Autodesk Inventor part; units mm, degrees
ref_plane "Work Plane1" through (29, 0, 0) normal (0, -1, 0) x (1, 0, 0)
ref_plane "YZ Plane" through (0, 0, 0) normal (1, 0, 0) x (0, 1, 0)
ref_plane "XZ Plane" through (0, 0, 0) normal (0, 1, 0) x (-1, 0, 0)
sketch "Szkic1" plane through (0, 0, 0) normal (0, 0, 1) x (1, 0, 0)
  line L0 (-1.1667, 0) -> (10, 0)
  line L1 (10, 0) -> (10, 2.5)
  line L2 (10, 2.5) -> (2, 2.5)
  line L3 (2, 2.5) -> (1.5091, 2.5)
  line L4 (1.5091, 2.5) -> (0, 2.5)
  line L5 (0, 2.5) -> (0, 4.25)
  line L6 (0, 4.25) -> (-5, 4.25)
  line L7 (-5, 4.25) -> (-5, 2.3094)
  line L8 (-5, 2.3094) -> (-2.5, 2.3094)
  line L9 (-2.5, 2.3094) -> (-1.1667, 0)
  line L10 (-8, 0) -> (13, 0)
  line L11 (0, -0.85) -> (0, 5.1)
  line L12 (2, 2.5) -> (0, 2.5) construction
  dimension "d1" = 8
  dimension "d2" = 0.4909
  dimension "d3" = 5
  dimension "d4" = 2.5
  dimension "d5" = 60
  dimension "d6" = 5
  dimension "d7" = 5
  dimension "d8" = 4.6188
  dimension "d9" = 8.5
  dimension "d26" = 10
revolve "Bryła" add sketch "Szkic1" angle 360 about axis through (-1.1667, 0, 0) along (1, 0, 0)
sketch "Szkic2" plane through (-5, 0, 0) normal (-1, 0, 0) x (0, 0, 1)
  circle A0 centre (0, 0) radius 2.3094
  line L0 (0, -5.95) -> (0, 5.95)
  line L1 (-5.95, 0) -> (5.95, 0)
  line L2 (2.3094, 0) -> (1.1547, -2)
  line L3 (1.1547, -2) -> (-1.1547, -2)
  line L4 (-1.1547, -2) -> (-2.3094, 0)
  line L5 (-2.3094, 0) -> (-1.1547, 2)
  line L6 (-1.1547, 2) -> (1.1547, 2)
  line L7 (1.1547, 2) -> (2.3094, 0)
extrude "Szczelina" add sketch "Szkic2" against normal up to next contours L7 A0 | A0 L2 | L6 L0 A0 | A0 L0 L3 | L0 L6 A0 | A0 L3 L0 | L4 A0 | A0 L5
fillet "Zaokrąglenie1" radius 0.5 1 edges at (-5, -4.25, 0)
thread "Gwint"
chamfer "Faza1" distance 0.4908 distance2 0.4908 1 edges at (10, -2.5, 0) measured on face at (10, -0.7741, -0.6858)
ref_plane "Work Plane1" through (29, 0, 0) normal (0, -1, 0) x (1, 0, 0)
fillet "Fillet2" radius 0.1 1 edges at (0, -2.5, 0)
equation "\"d1\" = GEL"
equation "\"d3\" = KOH"
equation "\"d4\" = INTI"
equation "\"d6\" = GD"
equation "\"d7\" = BDM"
equation "\"d8\" = 1.1547 * SW"
equation "\"d9\" = KOD"
equation "\"d26\" = NLG"
equation "\"d30\" = R"
equation "\"d17\" = RR"
equation "\"d13\" = GEL"
equation "\"d15\" = -0.5 * SPD + 0.5 * GD"
equation "\"d16\" = GUL"
equation "\"GD\" = NND"
equation "\"NLG\" = 10"
equation "\"GEL\" = 8"
equation "\"KOD\" = 8.5"
equation "\"KOH\" = NND"
equation "\"INTI\" = 2.5"
equation "\"GAL\" = 0.61345 * PTC"
equation "\"GUL\" = 0.61345 * PTC"
equation "\"BDM\" = NND"
equation "\"SW\" = 4"
equation "\"RR\" = 0.1 * NND"
equation "\"SPD\" = NND - 1.2269 * PTC"
equation "\"R\" = 0.1"
equation "\"PHH\" = 0.13"
equation "\"GD1\" = THREADDIA - 1.2269 * PTC"
equation "\"THREADDIA\" = 5"
equation "\"FAWI\" = 45deg"
equation "\"PTC\" = 0.8"
equation "\"KOH1\" = 4.5"
equation "\"NND\" = 5"
equation "\"TOA\" = 30deg"
equation "\"E0\" = 1.155 * SW"
properties part number "AS 1420 - 1973 - M5 x 10" material "Stal, miękka"
Read the model definition and answer for the solid it produces. Units are mm, in the model's axes. A direction names the side the tool comes from. Give positions to 0.01 mm unless a question says otherwise; leave off trailing zeros. Loops run counter-clockwise (first coordinate to the right, second up) from the corner with the lowest first, then second, coordinate; pieces in that order, holes last. Notation, with made-up numbers: (38.25, 54.5) - (63.25, 54.5) arc R18 cw to (63.25, 60.5) - close; hole circle Ø6 at (60.25, 66.5). An arc over 180 degrees is marked (long way). Answer as CSV lines item,"result". Start each with the question number.
1) Find section A-A (x = 8.5). Write down the section's boundary in (y, z), then the cut area to 3 significant figures.
2) Straight lines are drawn through the part: L1, parallel to X at y = 0, z = 3.25; L2, parallel to Z at x = 3.75, y = -1.5; L3, parallel to Y at x = -3, z = 1.25. For each, find the intervals that lie inside material, in ascending order. Write a range as from..to.
3) Determine the mould class of faces 1 (the face through (-2.282, 2.285, -3.584)), 2 (the face through (-5, -2, 2)), 3 (the face through (-3.68, -0.99, 1.74)) for opening direction Z: released by +Z, released by -Z, zero draft, split by the parting line, or undercut.
4) Which of the six approach directions +Z, -Z, +X, -X, +Y, -Y give full straight-line access (tool end or side, diameter ignored) to faces 4 (the face through (0, 2, 2)), 5 (the face through (-4, 2, 0)), 6 (the face through (10, 0, 0))?
5) Each of these flat-tipped pins is pushed along its axis until it touches: pin 1 Ø1 at (y, z) = (3, 3) entering from +X; pin 2 Ø1.5 at (y, z) = (0.5, 0) entering from -X; pin 3 Ø1.5 at (x, z) = (0, -1.5) entering from +Y. Where does it stop, or does it pass through?
Findings below:
1,outline,"circle Ø5 at (0, 0)"
1,area,"19.6 mm^2"
2,L1,"-5..0"
2,L2,"-2..2"
2,L3,"-4.06..-1.83, 1.83..4.06"
3,face 1,"split by the parting line"
3,face 2,"zero draft"
3,face 3,"undercut"
4,face 4,"+X"
4,face 5,"-X"
4,face 6,"+Z, -Z, +X, +Y, -Y"
5,pin 1,"x = 0"
5,pin 2,"x = -1.89"
5,pin 3,"y = 4.18"
